The model under review builds one solid part; all positions refer to its coordinate system, in mm. A direction names the side the tool comes from. Round coordinates to 2 decimals unless told otherwise and drop trailing zeros. Order: outer loops, then holes, each group sorted by start corner. A loop starts at its lowest first (then second) coordinate and runs counter-clockwise, first axis right, second up. Notation, with made-up numbers: M -4,29.25 L 4,29.25 A25 cw 4,68.25 Z; hole C 63,52.5 d4. An arc over 180 degrees is marked long. One line per item, written item: value. Start each with the question number.
from build123d import *

# Parameters (mm, degrees)
SKETCH1_W              = 25
SKETCH1_H              = 3.35
SKETCH1_R              = 1.025
STANDOFF_EXTRUDE_DEPTH = 11.24
SKETCH2_W              = 15.62
SKETCH2_H              = 7
STANDOFF_CUT_DEPTH     = 18.140889709
CHAMFER1_SIZE          = 6
FILLET2_R              = 0.6


with BuildPart() as part:
    # Sketch1 → Standoff Extrude (new body)
    with BuildSketch(Plane(origin=(0, 0, 0), x_dir=(1, 0, 0), z_dir=(0, 1, 0))):
        Rectangle(SKETCH1_W, SKETCH1_H)
        with Locations(Location((-10.25, 0, 0), (0, 0, 270))):
            Circle(SKETCH1_R, mode=Mode.SUBTRACT)
        with Locations(Location((10.25, 0, 0), (0, 0, 270))):
            Circle(SKETCH1_R, mode=Mode.SUBTRACT)
    extrude(amount=STANDOFF_EXTRUDE_DEPTH)

    # Sketch2 → Standoff Cut (cut, through all)
    with BuildSketch(Plane.XY.offset(1.675)):
        with Locations((0, 7.74)):
            Rectangle(SKETCH2_W, SKETCH2_H)
    extrude(amount=-STANDOFF_CUT_DEPTH, mode=Mode.SUBTRACT)

    # Chamfer1
    chamfer1_edges = [part.edges().sort_by_distance(p)[0] for p in [
        (-7.81, 4.24, 0),
        (7.81, 4.24, 0),
    ]]
    chamfer(chamfer1_edges, length=CHAMFER1_SIZE)

    # Fillet2
    fillet2_edges = [part.edges().sort_by_distance(p)[0] for p in [
        (12.5, 11.24, 0),
        (10.155, 11.24, -1.675),
        (-10.155, 11.24, -1.675),
        (10.155, 11.24, 1.675),
        (-7.81, 10.74, -1.675),
        (-7.81, 11.24, 0),
        (7.81, 11.24, 0),
        (-7.81, 10.74, 1.675),
        (7.81, 10.74, 1.675),
        (7.81, 10.74, -1.675),
        (0, 4.24, 1.675),
        (0, 4.24, -1.675),
        (-12.5, 11.24, 0),
        (4.81, 7.24, 1.675),
        (4.81, 7.24, -1.675),
        (-4.81, 7.24, 1.675),
        (-4.81, 7.24, -1.675),
        (0, 0, -1.675),
        (12.5, 0, 0),
        (0, 0, 1.675),
        (-12.5, 0, 0),
        (-10.155, 11.24, 1.675),
        (-12.5, 5.62, -1.675),
        (12.5, 5.62, -1.675),
        (12.5, 5.62, 1.675),
        (-12.5, 5.62, 1.675),
    ]]
    fillet(fillet2_edges, radius=FILLET2_R)


solid = part.part
Item 1: Clearance check with a flat-ended pin moving along its axis: P1, Ø1.2, axis at x = -10.25, z = 0, coming from the +Y side. State where the tip first meets the part, or that it passes through.
Item 2: Consider section B-B, the plane z = 0. Give the boundary of the cut face in (x, y) (3 decimals), then the cut area to 3 significant figures.
Item 3: Wall thickness on L1, parallel to X at y = 8.75, z = 0 (3 decimals); L2, parallel to X at y = 3.25, z = 0.7; L3, parallel to X at y = 5.25, z = 0 (3 decimals): over which ranges is each line inside the solid? List them lowest first.
Item 4: Machinability: for faces 4 (the cylindrical face through (-4.98, 7.16, 1.5)), 5 (the flat face through (4.77, 7.2, 0.02)), 6 (the cylindrical face through (4.887, 7.075, -1.495)), which of the approach directions +Z, -Z, +X, -X, +Y, -Y give a long, thin tool a straight path to every point of the face, cutting with its end or side? Answer none if there is none.
Item 5: Consider section C-C, the plane x = 10.25. Give the boundary of the cut face in (y, z) (3 decimals).
Item 6: Consider section D-D, the plane y = 5.75. Count the separate pieces of the cut face and the enclosed holes in it, then the cut area to 3 significant figures.
Item 7: Consider section A-A, the plane y = 1.25. Give the boundary of the cut face in (x, z) (3 decimals), then the cut area to 3 significant figures.
Item 8: The part is to be moulded in two halves that separate along X. For faces 1 (the flat face through (-12.5, 6, 0)), 2 (the flat face through (-9, 11.24, 0)), 3 (the flat face through (0, 4.24, 0)), say which applies: pulls with the +X half, pulls with the -X half, needs draft (parallel to the pull), parting line crosses it, or undercut.
Computed:
1. P1: passes through
2. outline: M -12.5,0.6 A0.6 ccw -11.9,0 L -11.275,0 L -11.275,11.24 L -11.9,11.24 A0.6 ccw -12.5,10.64 Z; M -9.225,0 L 9.225,0 L 9.225,11.24 L 8.41,11.24 A0.6 ccw 7.81,10.64 L 7.81,10.24 L 1.81,4.24 L -1.81,4.24 L -7.81,10.24 L -7.81,10.64 A0.6 ccw -8.41,11.24 L -9.225,11.24 Z; M 11.275,0 L 11.9,0 A0.6 ccw 12.5,0.6 L 12.5,10.64 A0.6 ccw 11.9,11.24 L 11.275,11.24 Z
2. area: 161 mm^2
3. L1: x = -12.5 to -11.275, -9.225 to -6.32, 6.32 to 9.225, 11.275 to 12.5
3. L2: x = -12.5 to -11, -9.5 to 9.5, 11 to 12.5
3. L3: x = -12.5 to -11.275, -9.225 to -2.82, 2.82 to 9.225, 11.275 to 12.5
4. face 4: +Z, +Y
4. face 5: +Z, -Z, +Y
4. face 6: -Z, +Y
5. outline: M 0,-1.075 A0.6 ccw 0.6,-1.675 L 10.64,-1.675 A0.6 ccw 11.24,-1.075 L 11.24,-1.025 L 0,-1.025 Z; M 0,1.025 L 11.24,1.025 L 11.24,1.075 A0.6 ccw 10.64,1.675 L 0.6,1.675 A0.6 ccw 0,1.075 Z
6. separate pieces: 2
6. enclosed holes: 2
6. area: 54.2 mm^2
7. outline: M -12.5,-1.075 A0.6 ccw -11.9,-1.675 L 11.9,-1.675 A0.6 ccw 12.5,-1.075 L 12.5,1.075 A0.6 ccw 11.9,1.675 L -11.9,1.675 A0.6 ccw -12.5,1.075 Z; hole C -10.25,0 d2.05; hole C 10.25,0 d2.05
7. area: 76.8 mm^2
8. face 1: pulls with the -X half
8. face 2: needs draft
8. face 3: undercut
